Can you work these out from the model? Positions are in its coordinate system, mm. Round coordinates to 2 decimals unless told otherwise and drop trailing zeros. Loops run counter-clockwise (first coordinate to the right, second up) from the corner with the lowest first, then second, coordinate; pieces in that order, holes last. Notation, with made-up numbers: M 52,78 L 77,78 A16 ccw 77,97 Z; hole C -39.75,16 d11. An arc over 180 degrees is marked long. Return JSON: item names as keys, results as strings.
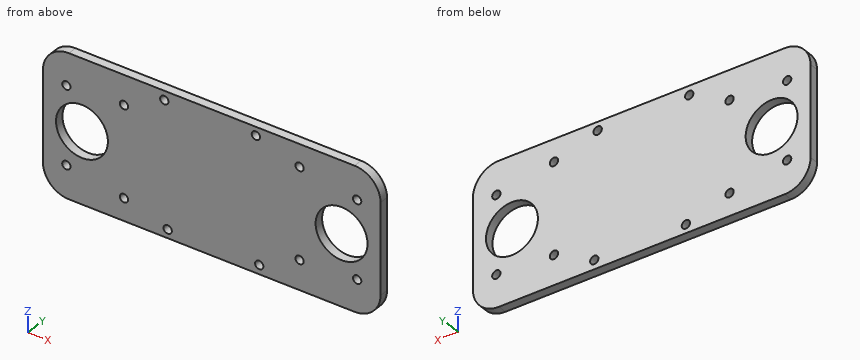
```python
from build123d import *

# Parameters (mm, degrees)
SKETCH1_W           = 130
SKETCH1_H           = 55
SKETCH1_R           = 1.6
SKETCH1_R_2         = 10
BOSS_EXTRUDE3_DEPTH = 3.5
FILLET3_R           = 10


with BuildPart() as part:
    # Sketch1 → Boss-Extrude3 (new body)
    with BuildSketch(Plane(origin=(0, 0, 0), x_dir=(1, 0, 0), z_dir=(0, 1, 0))):
        with Locations((65, -27.5)):
            Rectangle(SKETCH1_W, SKETCH1_H)
        with Locations((9, -12.5)):
            Circle(SKETCH1_R, mode=Mode.SUBTRACT)
        with Locations((9, -42.5)):
            Circle(SKETCH1_R, mode=Mode.SUBTRACT)
        with Locations((121, -42.5)):
            Circle(SKETCH1_R, mode=Mode.SUBTRACT)
        with Locations((121, -12.5)):
            Circle(SKETCH1_R, mode=Mode.SUBTRACT)
        with Locations((15, -27.5)):
            Circle(SKETCH1_R_2, mode=Mode.SUBTRACT)
        with Locations((115, -27.5)):
            Circle(SKETCH1_R_2, mode=Mode.SUBTRACT)
        with Locations((48.016852514, -3.3)):
            Circle(SKETCH1_R, mode=Mode.SUBTRACT)
        with Locations((46.716852514, -51.5)):
            Circle(SKETCH1_R, mode=Mode.SUBTRACT)
        with Locations((98.816852514, -46.4)):
            Circle(SKETCH1_R, mode=Mode.SUBTRACT)
        with Locations((98.816852514, -11.378935708)):
            Circle(SKETCH1_R, mode=Mode.SUBTRACT)
        with Locations((31.183147486, -43.621064292)):
            Circle(SKETCH1_R, mode=Mode.SUBTRACT)
        with Locations((31.183147486, -8.6)):
            Circle(SKETCH1_R, mode=Mode.SUBTRACT)
        with Locations((83.283147486, -3.5)):
            Circle(SKETCH1_R, mode=Mode.SUBTRACT)
        with Locations((81.983147486, -51.7)):
            Circle(SKETCH1_R, mode=Mode.SUBTRACT)
    extrude(amount=BOSS_EXTRUDE3_DEPTH)

    # Fillet3
    fillet3_edges = [part.edges().sort_by_distance(p)[0] for p in [
        (0, 1.75, 0),
        (130, 1.75, 0),
        (130, 1.75, 55),
        (0, 1.75, 55),
    ]]
    fillet(fillet3_edges, radius=FILLET3_R)


solid = part.part
```
Q1. Suppose I cut it at A-A, the plane z = 27.5. Please give me the cut outline in (x, y).
Results:
{"outline": "M 0,0 L 5,0 L 5,3.5 L 0,3.5 Z; M 25,0 L 105,0 L 105,3.5 L 25,3.5 Z; M 125,0 L 130,0 L 130,3.5 L 125,3.5 Z"}
Q2. Suppose I cut it at C-C, the plane z = 46.4. Please give me the cut outline in (x, y), plus the area to 3 significant figures.
Results:
{"outline": "M 0.1,0 L 97.22,0 L 97.22,3.5 L 0.1,3.5 Z; M 100.42,0 L 129.9,0 L 129.9,3.5 L 100.42,3.5 Z", "area": "443 mm2"}
Q3. Suppose I cut it at B-B, the plane x = 15. Please give me the cut outline in (y, z).
Results:
{"outline": "M 0,0 L 3.5,0 L 3.5,17.5 L 0,17.5 Z; M 0,37.5 L 3.5,37.5 L 3.5,55 L 0,55 Z"}
Q4. If I drill on line 1 along X through (y, z) = (1.5, 27.5); line 2 along X through (y, z) = (2.65, 51.5); line 3 along X through (y, z) = (1.9, 43), over which ranges is the centre line in solid material (lowest first)?
Results:
{"line 1": "x = 0 to 5, 25 to 105, 125 to 130", "line 2": "x = 2.4 to 45.12, 48.32 to 80.4, 83.57 to 127.6", "line 3": "x = 0 to 7.48, 10.52 to 29.71, 32.66 to 119.48, 122.52 to 130"}
Q5. I'm going to push a flat-ended pin straight in: pin 1 Ø2.5 at (x, z) = (121, 42.5) entering from +Y. Where does the tip first touch, or does it pass through?
Results:
{"pin 1": "passes through"}
